Here's how the part is built. I have some questions about the finished solid (model axes, mm). Face numbers are marked on the shaded views. A direction names the side the tool comes from. Give positions to 0.01 mm unless a question says otherwise; leave off trailing zeros. Loops run counter-clockwise (first coordinate to the right, second up) from the corner with the lowest first, then second, coordinate; pieces in that order, holes last.
Q1. For the marked faces 4, 5 and 6, which set-ups out of +Z, -Z, +X, -X, +Y, -Y let a thin tool reach every point of the face, with its end or its side?
Q2. If we section it at C-C (x = 17): Please give me the cut outline in (y, z).
Q3. If we section it at A-A (y = 26.25): Please give me the cut outline in (x, z).
Q4. If we section it at D-D (z = 27): Please give me the cut outline in (x, y), plus the area to 3 significant figures.
Q5. I need wall thicknesses on line 1 (X direction, y = 6.5, z = 42.5); line 2 (Z direction, x = -24.5, y = 1.75) (3 decimals); line 3 (Z direction, x = 16, y = 5.5). Which ranges of each line are inside material? Lowest first, please.
Q6. We'd pull the mould along X, two halves only. Please class the marked faces 1, 2 and 3: +X half, -X half, draft (parallel to the pull), parting line (faces both ways), or undercut.
Q7. Will these pins go through, and if not, where does the flat tip stop? P1, Ø2, axis at x = 0, z = 42.5, coming from the +Y side; P2, Ø12, axis at x = -7, y = 9.5, coming from the -Z side; P3, Ø8, axis at y = 19, z = 25.5, coming from the +X side; P4, Ø1, axis at y = 15, z = -17.5, coming from the +X side.
Q8. If we section it at B-B (z = 0): Please give me the cut outline in (x, y).
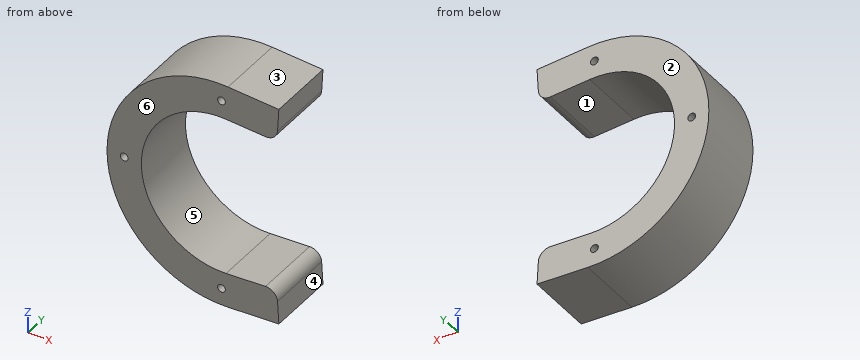
from build123d import *

# Parameters (mm, degrees)
SKETCH2_R           = 1.7
BOSS_EXTRUDE1_DEPTH = 29.5
FILLET2_R           = 5


with BuildPart() as part:
    # Sketch2 → Boss-Extrude1 (new body)
    with BuildSketch(Plane(origin=(0, 0, 0), x_dir=(1, 0, 0), z_dir=(0, 1, 0))):
        with BuildLine():
            Line((2.88691348, 49.91658773), (25.08691348, 48.632656232))
            Line((25.08691348, 48.632656232), (24.220839436, 33.657679913))
            Line((24.220839436, 33.657679913), (2.020839436, 34.941611411))
            ThreePointArc((2.020839436, 34.941611411), (-35, 0), (2.020839436, -34.941611411))
            Line((2.020839436, -34.941611411), (24.220839436, -33.657679913))
            Line((24.220839436, -33.657679913), (25.08691348, -48.632656232))
            Line((25.08691348, -48.632656232), (2.88691348, -49.91658773))
            ThreePointArc((2.88691348, -49.91658773), (-50, 0), (2.88691348, 49.91658773))
        make_face()
        with Locations(Location((-42.5, 0, 0), (0, 0, 270))):
            Circle(SKETCH2_R, mode=Mode.SUBTRACT)
        with Locations(Location((0, 42.5, 0), (0, 0, 270))):
            Circle(SKETCH2_R, mode=Mode.SUBTRACT)
        with Locations(Location((0, -42.5, 0), (0, 0, 90))):
            Circle(SKETCH2_R, mode=Mode.SUBTRACT)
    extrude(amount=BOSS_EXTRUDE1_DEPTH)

    # Fillet2
    fillet2_edges = [part.edges().sort_by_distance(p)[0] for p in [
        (24.220839436, 14.75, -33.657679913),
        (24.220839436, 14.75, 33.657679913),
    ]]
    fillet(fillet2_edges, radius=FILLET2_R)


solid = part.part
Check sheet entries:
1. face 4: +X, +Y, -Y
1. face 5: +Y, -Y
1. face 6: +Z, -Z, +X, -X, -Y
2. outline: (0, -49.1) - (29.5, -49.1) - (29.5, -34.08) - (0, -34.08) - close; (0, 34.08) - (29.5, 34.08) - (29.5, 49.1) - (0, 49.1) - close
3. outline: (2.02, -34.94) arc R35 cw (long way) to (2.02, 34.94) - (19.23, 33.95) arc R5 ccw to (24.51, 38.65) - (25.09, 48.63) - (2.89, 49.92) arc R50 ccw (long way) to (2.89, -49.92) - (25.09, -48.63) - (24.51, -38.65) arc R5 ccw to (19.23, -33.95) - close; hole circle Ø3.4 at (-42.5, 0); hole circle Ø3.4 at (0, -42.5); hole circle Ø3.4 at (0, 42.5)
4. outline: (-42.08, 0) - (-22.27, 0) - (-22.27, 29.5) - (-42.08, 29.5) - close
4. area: 584 mm2
5. line 1: x = -26.34 to -1.7, 1.7 to 24.73
5. line 2: z = -43.586 to -24.995, 24.995 to 43.586
5. line 3: z = -49.16 to -34.13, 34.13 to 49.16
6. face 1: undercut
6. face 2: draft
6. face 3: +X half
7. P1: passes through
7. P2: stops at z = -49.99
7. P3: stops at x = -18.83
7. P4: stops at x = -30.02
8. outline: (-50, 0) - (-44.2, 0) - (-44.2, 29.5) - (-50, 29.5) - close; (-40.8, 0) - (-35, 0) - (-35, 29.5) - (-40.8, 29.5) - close
